The model under review builds one solid part; all positions refer to its coordinate system, in mm. Face numbers are marked on the shaded views. A direction names the side the tool comes from. Coordinates: 2 decimals unless noted, no trailing zeros. Order: outer loops, then holes, each group sorted by start corner. A loop starts at its lowest first (then second) coordinate and runs counter-clockwise, first axis right, second up. Notation, with made-up numbers: (-23, -6.75) -> (6, -6.75) arc R37 cw to (6, 29.25) -> close; hole circle Ø9 at (86.5, 16). An arc over 180 degrees is marked (long way). Put each result on its own line as item: value.
Solid Edge part; units mm, degrees
sketch "Sketch1" plane through (0, 0, 0) normal (0, 0, 1) x (1, 0, 0)
  line L0 (-45, -22.5) -> (45, -22.5)
  line L1 (45, 22.5) -> (-45, 22.5)
  arc A0 (45, 22.5) -> (45, -22.5) centre (45, 0) cw
  arc A1 (-45, -22.5) -> (-45, 22.5) centre (-45, 0) cw
  circle A2 centre (-45, 0) radius 10
  circle A3 centre (45, 0) radius 10
extrude "Protrusion1" add sketch "Sketch1" along normal blind 15
sketch "Sketch2" plane through (0, -22.5, 7.5) normal (0, -1, 0) x (1, 0, 0)
  line L0 (15, 92.5) -> (-15, 92.5)
  line L1 (-15, 92.5) -> (-15, 62.5)
  line L2 (-15, 62.5) -> (15, 62.5)
  line L3 (15, 62.5) -> (15, 92.5)
  line L4 (10, 87.5) -> (-10, 87.5)
  line L5 (-10, 87.5) -> (-10, 67.5)
  line L6 (-10, 67.5) -> (10, 67.5)
  line L7 (10, 67.5) -> (10, 87.5)
extrude "ExtrudedProtrusion_2" add sketch "Sketch2" against normal blind 30
sketch "Sketch3" plane through (0, -12.5, 7.5) normal (0, -1, 0) x (1, 0, 0)
  line L0 (-40, 89.5) -> (-18, 89.5)
  arc A0 (-18, 89.5) -> (-15, 92.5) centre (-18, 92.5) ccw
  line L1 (-15, 62.5) -> (-15, 92.5)
  arc A1 (-18, 65.5) -> (-15, 62.5) centre (-18, 62.5) cw
  line L2 (-40, 65.5) -> (-18, 65.5)
  arc A2 (-40, 65.5) -> (-40, 89.5) centre (-40, 77.5) cw
  circle A3 centre (-40, 77.5) radius 5
extrude "ExtrudedProtrusion_3" add sketch "Sketch3" against normal blind 10
sketch "Sketch4" plane through (0, 0, 0) normal (0, -1, 0) x (1, 0, 0)
  line L0 (-24.5, 15) -> (-15, 70)
  line L1 (-15, 70) -> (0, 70)
  line L2 (0, 70) -> (0, 15)
  line L3 (0, 15) -> (-24.5, 15)
extrude "Protrusion2" add sketch "Sketch4" along normal up to vertex (22.5 mm away)
mirror "Mirror1" about plane through (0, 0, 0) normal (1, 0, 0) of "Protrusion2", "ExtrudedProtrusion_3"
sketch "Sketch5" plane through (0, 0, 0) normal (1, 0, 0) x (0, 1, 0)
  line L0 (22.5, 15) -> (7.5, 70)
  line L1 (7.5, 70) -> (0, 70)
  line L2 (0, 70) -> (0, 15)
  line L3 (0, 15) -> (22.5, 15)
extrude "ExtrudedProtrusion_9" add sketch "Sketch5" along normal mid plane 15
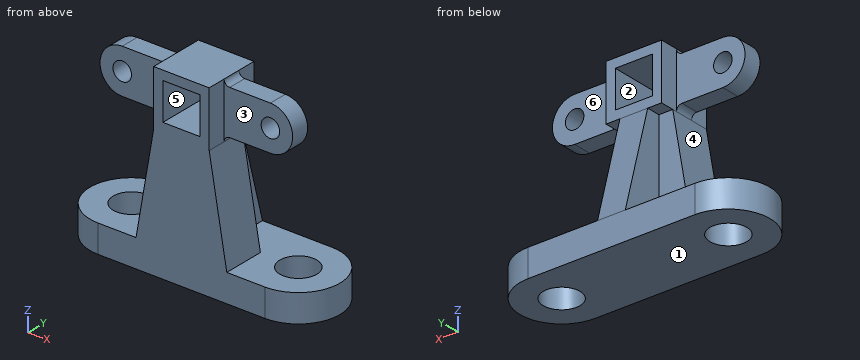
Item 1: Mouldability with a two-part tool opening along Z and no side actions: class the marked faces 1, 2 and 3 as +Z half, -Z half, draft (parallel to the pull), parting line (faces both ways), or undercut.
Answers below:
face 1: -Z half
face 2: undercut
face 3: draft
Item 2: Consider section A-A on z = 85. Write out the cut boundary in (x, y).
Answers below:
outline: (-52, -12.5) -> (-45, -12.5) -> (-45, -2.5) -> (-52, -2.5) -> close; (-35, -12.5) -> (-15, -12.5) -> (-15, -22.5) -> (-10, -22.5) -> (-10, 7.5) -> (-15, 7.5) -> (-15, -2.5) -> (-35, -2.5) -> close; (10, -22.5) -> (15, -22.5) -> (15, -12.5) -> (35, -12.5) -> (35, -2.5) -> (15, -2.5) -> (15, 7.5) -> (10, 7.5) -> close; (45, -12.5) -> (52, -12.5) -> (52, -2.5) -> (45, -2.5) -> close
Item 3: For pin 1 Ø8 at (y, z) = (-8.5, 52.5) entering from -X; pin 2 Ø6 at (y, z) = (0, 82.5) entering from -X; pin 3 Ø5 at (x, y) = (-50.5, 9) entering from +Z; pin 4 Ø8 at (x, z) = (-40, 84.5) entering from -Y, all flat-tipped, find the tip position at first contact; note any pin that passes through.
Answers below:
pin 1: x = -18.71
pin 2: x = -51.97
pin 3: z = 15
pin 4: through
Item 4: Consider section C-C on y = -7. Count the separate pieces of the cut face and the enclosed holes in it, and give its area (3 significant figures).
Answers below:
separate pieces: 3
enclosed holes: 3
area: 5,740 mm^2
Item 5: Consider section B-B on y = 6. Write out the cut boundary in (x, z).
Answers below:
outline: (-66.69, 0) -> (-53, 0) -> (-53, 15) -> (-66.69, 15) -> close; (-37, 0) -> (37, 0) -> (37, 15) -> (7.5, 15) -> (7.5, 70) -> (15, 70) -> (15, 100) -> (-15, 100) -> (-15, 70) -> (-7.5, 70) -> (-7.5, 15) -> (-37, 15) -> close; (53, 0) -> (66.69, 0) -> (66.69, 15) -> (53, 15) -> close; hole (-10, 75) -> (10, 75) -> (10, 95) -> (-10, 95) -> close
Item 6: For the marked faces 4, 5 and 6, list the 3-axis set-ups (+Z, -Z, +X, -X, +Y, -Y) from which the entire face can be reached by the end or side of a thin tool; tool diameter is ignored.
Answers below:
face 4: -X, +Y, -Y
face 5: +Y, -Y
face 6: +Z, +X, +Y
Item 7: Consider section D-D on z = 10.5. Write out the cut boundary in (x, y), and give its area (3 significant figures).
Answers below:
outline: (-45, -22.5) -> (45, -22.5) arc R22.5 ccw to (45, 22.5) -> (-45, 22.5) arc R22.5 ccw to start; hole circle Ø20 at (-45, 0); hole circle Ø20 at (45, 0)
area: 5,010 mm^2
Item 8: For line 1 (Z direction, x = -40, y = -6.25); line 2 (Z direction, x = -40, y = -9.5); line 3 (Y direction, x = -45, z = 12), list the stretches that pass through material, from the lowest coordinate up. Write a range as from..to.
Answers below:
line 1: 73..80, 90..97
line 2: 0..15, 73..80, 90..97
line 3: -22.5..-10, 10..22.5
